Could you check a few things on this model? Use its own coordinates, in mm. Give positions to 0.01 mm unless a question says otherwise; leave off trailing zeros. Order: outer loops, then holes, each group sorted by start corner. A loop starts at its lowest first (then second) coordinate and runs counter-clockwise, first axis right, second up. Notation, with made-up numbers: (12.5, 52.5) - (21.5, 52.5) arc R14 ccw to (21.5, 74.5) - close; hole circle Ø7 at (-15.5, 0.25). An arc over 180 degrees is marked (long way). One line per question, with ' | ' between items. Start each with the question number.
1. Imagine slicing it at A-A (z = 4.25). Please give me the cut outline in (x, y), and give its area (3 significant figures).
2. Imagine slicing it at B-B (x = 132). Please give me the cut outline in (y, z).
3. For P1, Ø4, axis at x = 19.5, y = 5, coming from the -Z side; P2, Ø3, axis at y = -51.5, z = 11, coming from the +X side; P3, Ø0.6, axis at x = 85.5, z = 1.5, coming from the -Y side; P4, Ø2, axis at x = 29, z = 1.5, coming from the -Y side, each with a flat end and sliding along its axis, tell me the tip position at first contact or that it passes through.
4. Imagine slicing it at C-C (x = 52). Please give me the cut outline in (y, z).
5. I need wall thicknesses on probe 1 along Y at (x, z) = (49.5, 3.5); probe 2 along Y at (x, z) = (136.5, 5.25); probe 3 along X at (y, z) = (-101, 5.5). Which ranges of each line are inside material? Lowest first, please. Write a range as from..to.
```python
from build123d import *

# Parameters (mm, degrees)
BOSS_EXTRUDE1_DEPTH = 15
FILLET1_R           = 10
FILLET2_R           = 10
FILLET4_R           = 10
FILLET5_R           = 10
FILLET6_R           = 10
CUT_EXTRUDE1_DEPTH  = 2


with BuildPart() as part:
    # Sketch1 → Boss-Extrude1 (new body)
    with BuildSketch(Plane.XY):
        Polygon((0, 103.5), (0, -103.5), (75, -121.5), (150, -46.5), (150, 103.5), align=None)
    extrude(amount=BOSS_EXTRUDE1_DEPTH)

    # Fillet1
    fillet1_edges = [part.edges().sort_by_distance(p)[0] for p in [
        (0, -103.5, 7.5),
    ]]
    fillet(fillet1_edges, radius=FILLET1_R)

    # Fillet2
    fillet2_edges = [part.edges().sort_by_distance(p)[0] for p in [
        (75, -121.5, 7.5),
    ]]
    fillet(fillet2_edges, radius=FILLET2_R)

    # Fillet4
    fillet4_edges = [part.edges().sort_by_distance(p)[0] for p in [
        (150, -46.5, 7.5),
    ]]
    fillet(fillet4_edges, radius=FILLET4_R)

    # Fillet5
    fillet5_edges = [part.edges().sort_by_distance(p)[0] for p in [
        (150, 103.5, 7.5),
    ]]
    fillet(fillet5_edges, radius=FILLET5_R)

    # Fillet6
    fillet6_edges = [part.edges().sort_by_distance(p)[0] for p in [
        (0, 103.5, 7.5),
    ]]
    fillet(fillet6_edges, radius=FILLET6_R)

    # Sketch2 → Cut-Extrude1 (cut)
    with BuildSketch(Plane(origin=(0, 0, 0), x_dir=(-1, 0, 0), z_dir=(0, 0, -1))):
        Polygon((-12.235489358, 0), (-12.235489358, 3.562429258), (-83.581556078, 94.421338251), (-87.783155362, 94.421338251), (-87.783155362, 3.562429258), (-87.783155362, 0), (-83.581556078, 0), (-46.597715557, 0), (-42.603563367, 0), align=None)
        Polygon((-46.597715557, 3.562429258), (-83.581556078, 3.562429258), (-83.581556078, 89.170075728), (-46.597715557, 42.94675871), align=None, mode=Mode.SUBTRACT)
        Polygon((-42.603563367, 37.954768687), (-15.085832519, 3.562429258), (-42.603563367, 3.562429258), align=None, mode=Mode.SUBTRACT)
    extrude(amount=-CUT_EXTRUDE1_DEPTH, mode=Mode.SUBTRACT)


solid = part.part
```
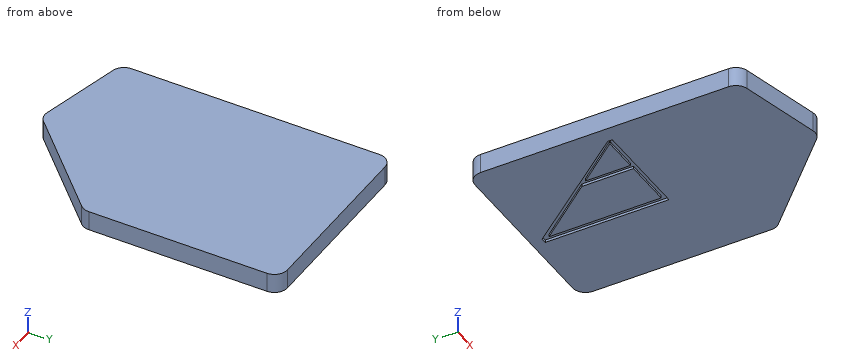
Results found:
1) outline: (0, -95.62) arc R10 ccw to (7.67, -105.34) - (69.55, -120.19) arc R10 ccw to (78.96, -117.54) - (147.07, -49.43) arc R10 ccw to (150, -42.36) - (150, 93.5) arc R10 ccw to (140, 103.5) - (10, 103.5) arc R10 ccw to (0, 93.5) - close | area: 30,200 mm2
2) outline: (-64.5, 0) - (103.5, 0) - (103.5, 15) - (-64.5, 15) - close
3) P1: stops at z = 0 | P2: stops at x = 146.5 | P3: stops at y = -111.3 | P4: stops at y = -110.7
4) outline: (-115.98, 0) - (0, 0) - (0, 2) - (3.56, 2) - (3.56, 0) - (49.7, 0) - (49.7, 2) - (54.2, 2) - (54.2, 0) - (103.5, 0) - (103.5, 15) - (-115.98, 15) - close
5) probe 1: y = -115.38..103.5 | probe 2: y = -60..103.5 | probe 3: x = 1.57..95.5
